```python
from build123d import *

# Parameters (mm, degrees)
SKETCH2_W           = 412.75
SKETCH2_H           = 444.5
BOSS_EXTRUDE1_DEPTH = 69.85
SHELL1_T            = -1.5875
SKETCH4_W           = 127
SKETCH4_H           = 412.75
CUT_EXTRUDE1_DEPTH  = 69.85


with BuildPart() as part:
    # Sketch2 → Boss-Extrude1 (new body)
    with BuildSketch(Plane.XY):
        with Locations((87.819148936, -186.024601064)):
            Rectangle(SKETCH2_W, SKETCH2_H)
    extrude(amount=BOSS_EXTRUDE1_DEPTH)

    # Shell1
    shell1_openings = [part.faces().sort_by_distance(p)[0] for p in [
        (87.819148936, 36.225398936, 34.925),
    ]]
    offset(amount=SHELL1_T, openings=shell1_openings, kind=Kind.INTERSECTION)

    # Sketch4 → Cut-Extrude1 (cut)
    with BuildSketch(Plane.XY.offset(69.85)):
        with Locations((93.402369386, -170.125111794)):
            Rectangle(SKETCH4_W, SKETCH4_H)
    extrude(amount=-CUT_EXTRUDE1_DEPTH, mode=Mode.SUBTRACT)


solid = part.part
```
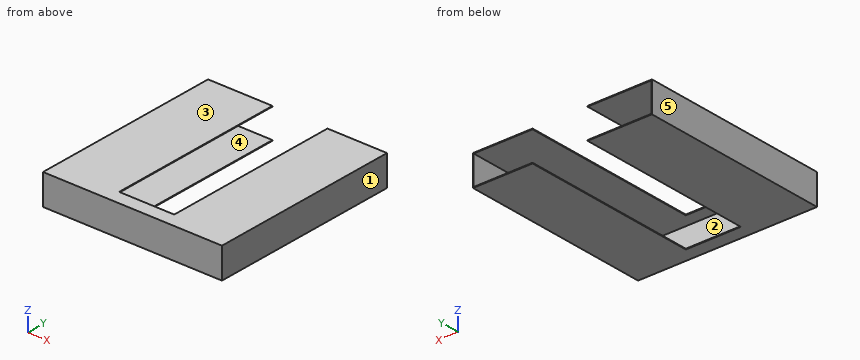
Read the model definition and answer for the solid it produces. Units are mm, in the model's axes. Face numbers are marked on the shaded views. A direction names the side the tool comes from. Round coordinates to 2 decimals unless told otherwise and drop trailing zeros. Write each loop counter-clockwise with the first axis right and the second up, starting at its lowest first coordinate (ties: lowest second). Pieces come first, ordered by that corner, then holes. Notation, with made-up numbers: (86.25, 16) -> (112.25, 16) arc R26 ccw to (112.25, 53) -> close; hole circle Ø4 at (-34.5, -8). An arc over 180 degrees is marked (long way). Answer in a Markdown table with one row per item. Add a question column.
1) Given P1, Ø1.5, axis at x = -51.5, z = 20, coming from the +Y side; P2, Ø0.8, axis at x = 93, z = 0.5, coming from the +Y side, each flat-ended and moving along its own axis, determine where each tip first touches the part or whether it passes through.
2) Consider line 1 (X direction, y = -112, z = 4); line 2 (Z direction, x = 158, y = 2.5); line 3 (Y direction, x = -41.5, z = 62). Determine where each line is inside the solid, lowest interval first.
3) Determine the mould class of the marked faces 3, 4 and 5 for opening direction Z: pulls with the +Z half, pulls with the -Z half, needs draft (parallel to the pull), parting line crosses it, or undercut.
4) Which of the six approach directions +Z, -Z, +X, -X, +Y, -Y give full straight-line access (tool end or side, diameter ignored) to the marked faces 1 and 2?
5) Find section A-A, the plane y = -279. Determine the outline of the cut face in (x, z), and give its area (3 significant figures).
6) Find section B-B, the plane z = 28.5. Determine the outline of the cut face in (x, y).
7) Find section C-C, the plane x = -69. Determine the outline of the cut face in (y, z).
Findings below:
| question | item | result |
|---|---|---|
| 1 | P1 | y = -406.69 |
| 1 | P2 | y = -376.5 |
| 2 | line 1 | -118.56 to -116.97, 292.61 to 294.19 |
| 2 | line 2 | 0 to 1.59, 68.26 to 69.85 |
| 2 | line 3 | -408.27 to -406.69 |
| 3 | face 3 | pulls with the +Z half |
| 3 | face 4 | undercut |
| 3 | face 5 | needs draft |
| 4 | face 1 | +Z, -Z, +X, +Y, -Y |
| 4 | face 2 | +Y |
| 5 | outline | (-118.56, 0) -> (29.9, 0) -> (29.9, 1.59) -> (-116.97, 1.59) -> (-116.97, 68.26) -> (29.9, 68.26) -> (29.9, 69.85) -> (-118.56, 69.85) -> close; (156.9, 0) -> (294.19, 0) -> (294.19, 69.85) -> (156.9, 69.85) -> (156.9, 68.26) -> (292.61, 68.26) -> (292.61, 1.59) -> (156.9, 1.59) -> close |
| 5 | area | 1,120 mm² |
| 6 | outline | (-118.56, -408.27) -> (294.19, -408.27) -> (294.19, 36.23) -> (292.61, 36.23) -> (292.61, -406.69) -> (-116.97, -406.69) -> (-116.97, 36.23) -> (-118.56, 36.23) -> close |
| 7 | outline | (-408.27, 0) -> (36.23, 0) -> (36.23, 1.59) -> (-406.69, 1.59) -> (-406.69, 68.26) -> (36.23, 68.26) -> (36.23, 69.85) -> (-408.27, 69.85) -> close |
